```python
from build123d import *

# Parameters (mm, degrees)
SKETCH2_W           = 0.5
SKETCH2_H           = 24.3
SKETCH2_H_2         = 25.6
SKETCH2_H_3         = 24.7
SKETCH2_H_4         = 23.7
SKETCH2_W_2         = 0.65
SKETCH2_H_5         = 1.7
BOSS_EXTRUDE1_DEPTH = 0.2
CUT_EXTRUDE1_DEPTH  = 27.6


with BuildPart() as part:
    # Sketch1 → Revolve1 (revolve)
    with BuildSketch(Plane.XY):
        with BuildLine():
            Line((0, 0), (2.75, 0))
            Line((2.75, 0), (2.75, 1))
            Line((2.75, 1), (2.375, 1))
            Line((2.375, 1), (2.375, 6.225))
            ThreePointArc((2.375, 6.225), (1.679378605, 7.904378605), (0, 8.6))
            Line((0, 8.6), (0, 0))
        make_face()
    revolve(axis=Axis((0, 0, 0), (0, -1, 0)))

    # Sketch2 → Boss-Extrude1 (add, symmetric)
    with BuildSketch(Plane.XY):
        with Locations((1.95, -12.15)):
            Rectangle(SKETCH2_W, SKETCH2_H)
        with Locations((0.65, -12.8)):
            Rectangle(SKETCH2_W, SKETCH2_H_2)
        with Locations((-0.65, -12.35)):
            Rectangle(SKETCH2_W, SKETCH2_H_3)
        with Locations((-1.95, -11.85)):
            Rectangle(SKETCH2_W, SKETCH2_H_4)
        with Locations((-1.95, -3.85)):
            Rectangle(SKETCH2_W_2, SKETCH2_H_5)
        with Locations((-0.65, -3.85)):
            Rectangle(SKETCH2_W_2, SKETCH2_H_5)
        with Locations((0.65, -3.85)):
            Rectangle(SKETCH2_W_2, SKETCH2_H_5)
        with Locations((1.95, -3.85)):
            Rectangle(SKETCH2_W_2, SKETCH2_H_5)
    extrude(amount=BOSS_EXTRUDE1_DEPTH, both=True)

    # Sketch3 → Cut-Extrude1 (cut, through all)
    with BuildSketch(Plane(origin=(0, 1, 0), x_dir=(1, 0, 0), z_dir=(0, 1, 0))):
        Polygon((2.375, 24.558218042), (2.375, 1.386317063), (2.375, -1.386317063), (2.375, -24.558218042), (48.718801957, -24.558218042), (48.718801957, 24.558218042), align=None)
    extrude(amount=-CUT_EXTRUDE1_DEPTH, mode=Mode.SUBTRACT)


solid = part.part
```
Geometry check sheet. Reference: the model listing, model coordinates, mm. A direction names the side the tool comes from. Coordinates: 2 decimals unless noted, no trailing zeros. Order: outer loops, then holes, each group sorted by start corner. A loop starts at its lowest first (then second) coordinate and runs counter-clockwise, first axis right, second up. Notation, with made-up numbers: (83.25, 30.25) - (105.25, 30.25) arc R31 cw to (105.25, 65.25) - close; hole circle Ø3 at (60, -39). An arc over 180 degrees is marked (long way). Answer in a Markdown table with one row per item. Add a question column.
1. Gauge pin test, flat ends, axial feed: pin 1 Ø1.5 at (x, z) = (-1, -1.5) entering from -Y; pin 2 Ø2 at (x, z) = (-2, 1) entering from +Y; pin 3 Ø1 at (x, z) = (-1.5, 1) entering from +Y. Record the tip position at first contact, or that the pin passes through.
2. Section check D-D (y = 3.5). Enter the section's corners in (x, z) (3 decimals).
3. Access from +Z, -Z, +X, -X, +Y, -Y to the whole of each face (thin tool, end or side, straight path). Record for faces 1 (the face through (1.096, 3.649, -2.107)), 2 (the face through (2.375, 0.5, 0)).
4. Section check C-C (z = -1). Enter the section's corners in (x, y) (3 decimals), plus the area to 3 significant figures.
5. Section check B-B (x = 0). Enter the section's corners in (y, z) (3 decimals), plus the area to 3 significant figures.
6. Section check A-A (y = -18.5). Enter the section's corners in (x, z).
7. Material ranges on L1, parallel to Z at x = -0.6, y = -4; L2, parallel to Y at x = -2.1, z = 1.55; L3, parallel to Y at x = -0.2, z = 2.1, recorded low to high. Write a range as [from, to].
Data:
| question | item | result |
|---|---|---|
| 1 | pin 1 | stops at y = 0 |
| 1 | pin 2 | stops at y = 8.25 |
| 1 | pin 3 | stops at y = 8.21 |
| 2 | outline | circle Ø4.75 at (0, 0) |
| 3 | face 1 | +Y |
| 3 | face 2 | +Z, -Z, +X, +Y, -Y |
| 4 | outline | (-2.562, 0) - (2.375, 0) - (2.375, 1) - (2.154, 1) - (2.154, 6.225) arc R2.154 ccw to (-2.154, 6.225) - (-2.154, 1) - (-2.562, 1) - close |
| 4 | area | 34.7 mm² |
| 5 | outline | (0, -2.75) - (1, -2.75) - (1, -2.375) - (6.225, -2.375) arc R2.375 ccw to (6.225, 2.375) - (1, 2.375) - (1, 2.75) - (0, 2.75) - close |
| 5 | area | 39.2 mm² |
| 6 | outline | (-2.2, -0.2) - (-1.7, -0.2) - (-1.7, 0.2) - (-2.2, 0.2) - close; (-0.9, -0.2) - (-0.4, -0.2) - (-0.4, 0.2) - (-0.9, 0.2) - close; (0.4, -0.2) - (0.9, -0.2) - (0.9, 0.2) - (0.4, 0.2) - close; (1.7, -0.2) - (2.2, -0.2) - (2.2, 0.2) - (1.7, 0.2) - close |
| 7 | L1 | z = [-0.2, 0.2] |
| 7 | L2 | y = [0, 1] |
| 7 | L3 | y = [0, 7.32] |
